from build123d import *

# Parameters (mm, degrees)
BOSS_EXTRUDE1_DEPTH = 10
FILLET1_R           = 5
SKETCH2_R           = 1.75
CUT_EXTRUDE1_DEPTH  = 15
SKETCH3_R           = 1.75
CUT_EXTRUDE2_DEPTH  = 15
SKETCH4_R           = 3.25
CUT_EXTRUDE3_DEPTH  = 3


with BuildPart() as part:
    # Sketch1 → Boss-Extrude1 (new body)
    with BuildSketch(Plane(origin=(0, 0, 0), x_dir=(1, 0, 0), z_dir=(0, 1, 0))):
        Polygon((6, 6), (30, 6), (30, -6), (6, -6), (6, -30), (-6, -30), (-6, -6), (-30, -6), (-30, 6), (-6, 6), (-6, 30), (6, 30), align=None)
    extrude(amount=BOSS_EXTRUDE1_DEPTH)

    # Fillet1
    fillet1_edges = [part.edges().sort_by_distance(p)[0] for p in [
        (30, 5, -6),
        (30, 5, 6),
        (6, 5, 30),
        (-6, 5, 30),
        (-30, 5, 6),
        (-30, 5, -6),
        (-6, 5, -30),
        (6, 5, -30),
    ]]
    fillet(fillet1_edges, radius=FILLET1_R)

    # Sketch2 → Cut-Extrude1 (cut)
    with BuildSketch(Plane(origin=(0, 10, 0), x_dir=(1, 0, 0), z_dir=(0, 1, 0))):
        with Locations(Location((-8, 0, 0), (0, 0, 270))):
            Circle(SKETCH2_R)
        with Locations(Location((8, 0, 0), (0, 0, 270))):
            Circle(SKETCH2_R)
        with Locations(Location((0, 9.5, 0), (0, 0, 270))):
            Circle(SKETCH2_R)
        with Locations(Location((0, -9.5, 0), (0, 0, 270))):
            Circle(SKETCH2_R)
    extrude(amount=-CUT_EXTRUDE1_DEPTH, mode=Mode.SUBTRACT)

    # Sketch3 → Cut-Extrude2 (cut)
    with BuildSketch(Plane(origin=(0, 10, 0), x_dir=(1, 0, 0), z_dir=(0, 1, 0))):
        with Locations(Location((0, 24, 0), (0, 0, 270))):
            Circle(SKETCH3_R)
        with Locations(Location((24, 0, 0), (0, 0, 270))):
            Circle(SKETCH3_R)
        with Locations(Location((-24, 0, 0), (0, 0, 270))):
            Circle(SKETCH3_R)
        with Locations(Location((0, -24, 0), (0, 0, 270))):
            Circle(SKETCH3_R)
    extrude(amount=-CUT_EXTRUDE2_DEPTH, mode=Mode.SUBTRACT)

    # Sketch4 → Cut-Extrude3 (cut)
    with BuildSketch(Plane.XZ):
        with Locations(Location((0, -9.5, 0), (0, 0, 270))):
            Circle(SKETCH4_R)
        with Locations(Location((-8, 0, 0), (0, 0, 270))):
            Circle(SKETCH4_R)
        with Locations(Location((8, 0, 0), (0, 0, 270))):
            Circle(SKETCH4_R)
        with Locations(Location((0, 9.5, 0), (0, 0, 270))):
            Circle(SKETCH4_R)
    extrude(amount=-CUT_EXTRUDE3_DEPTH, mode=Mode.SUBTRACT)


solid = part.part
Could you check a few things on this model? Use its own coordinates, in mm. A direction names the side the tool comes from. Round coordinates to 2 decimals unless told otherwise and drop trailing zeros. Write each loop counter-clockwise with the first axis right and the second up, starting at its lowest first coordinate (ties: lowest second). Pieces come first, ordered by that corner, then holes. Notation, with made-up numbers: (22.25, -17) - (76.25, -17) arc R19 ccw to (76.25, 12) - close; hole circle Ø6 at (-15.75, -11). An arc over 180 degrees is marked (long way). Put each result on its own line as item: value. Start each with the question number.
(1) For faces 4 (the flat face through (-9.4, 3, -1.4)), 5 (the flat face through (-15, 5, 6)), 6 (the cylindrical face through (9.735, 6.549, -0.228)), which set-ups out of +Z, -Z, +X, -X, +Y, -Y let a thin tool reach every point of the face, with its end or its side?
(2) I need wall thicknesses on probe 1 along X at (y, z) = (5, 0); probe 2 along X at (y, z) = (2.1, 9.5); probe 3 along X at (y, z) = (4.5, 24). Which ranges of each line are inside material? Lowest first, please.
(3) I want a section at A-A, the plane z = 24. Please give me the cut outline in (x, y).
(4) Thinking about a two-plate mould opening in X: for faces 1 (the flat face through (6, 5, 15)), 2 (the flat face through (0, 5, -30)), 3 (the cylindrical face through (-9.55, 6.55, 0.81)), which applies, released by +X, released by -X, zero draft, split by the parting line, or undercut?
(5) I want a section at B-B, the plane y = 8. Give the number of separate pieces and of enclosed holes in the cut face, plus the area to 3 significant figures.
(6) Will these pins go through, and if not, where does the flat tip stop? pin 1 (3 mm diameter, centred on x = 8, z = 0, fed in from -Y) (1 decimal); pin 2 (3 mm diameter, centred on y = 4, z = -13, fed in from +X); pin 3 (6 mm diameter, centred on x = 0, z = -9.5, fed in from -Y); pin 4 (4 mm diameter, centred on x = -21, y = 4.5, fed in from +Z).
(7) I want a section at D-D, the plane z = 0. Please give me the cut outline in (x, y).
(8) I want a section at C-C, the plane x = 24. Please give me the cut outline in (y, z), plus the area to 3 significant figures.
Here are the results:
1. face 4: -Y
1. face 5: +Z, -X, +Y, -Y
1. face 6: +Y, -Y
2. probe 1: x = -30 to -25.75, -22.25 to -9.75, -6.25 to 6.25, 9.75 to 22.25, 25.75 to 30
2. probe 2: x = -6 to -3.25, 3.25 to 6
2. probe 3: x = -6 to -1.75, 1.75 to 6
3. outline: (-6, 0) - (-1.75, 0) - (-1.75, 10) - (-6, 10) - close; (1.75, 0) - (6, 0) - (6, 10) - (1.75, 10) - close
4. face 1: released by +X
4. face 2: zero draft
4. face 3: undercut
5. separate pieces: 1
5. enclosed holes: 8
5. area: 1,180 mm^2
6. pin 1: passes through
6. pin 2: stops at x = 6
6. pin 3: stops at y = 3
6. pin 4: stops at z = 6
7. outline: (-30, 0) - (-25.75, 0) - (-25.75, 10) - (-30, 10) - close; (-22.25, 0) - (-11.25, 0) - (-11.25, 3) - (-9.75, 3) - (-9.75, 10) - (-22.25, 10) - close; (-6.25, 3) - (-4.75, 3) - (-4.75, 0) - (4.75, 0) - (4.75, 3) - (6.25, 3) - (6.25, 10) - (-6.25, 10) - close; (9.75, 3) - (11.25, 3) - (11.25, 0) - (22.25, 0) - (22.25, 10) - (9.75, 10) - close; (25.75, 0) - (30, 0) - (30, 10) - (25.75, 10) - close
8. outline: (0, -6) - (10, -6) - (10, -1.75) - (0, -1.75) - close; (0, 1.75) - (10, 1.75) - (10, 6) - (0, 6) - close
8. area: 85.0 mm^2
